Answer from the drawing. Dimensions are ordinates in mm from the lowest x, y and z of the part. Coordinates: 2 decimals unless noted, no trailing zeros. Write each loop counter-clockwise with the first axis right and the second up, starting at its lowest first coordinate (ties: lowest second). Pieces come first, ordered by that corner, then holes. Notation, with made-up numbers: (-38.75, 56) -> (-27.75, 56) arc R13 cw to (-27.75, 61) -> close; hole circle Ø6 at (-16, -10). An arc over 180 degrees is marked (long way). Return JSON: item names as keys, results as strings.
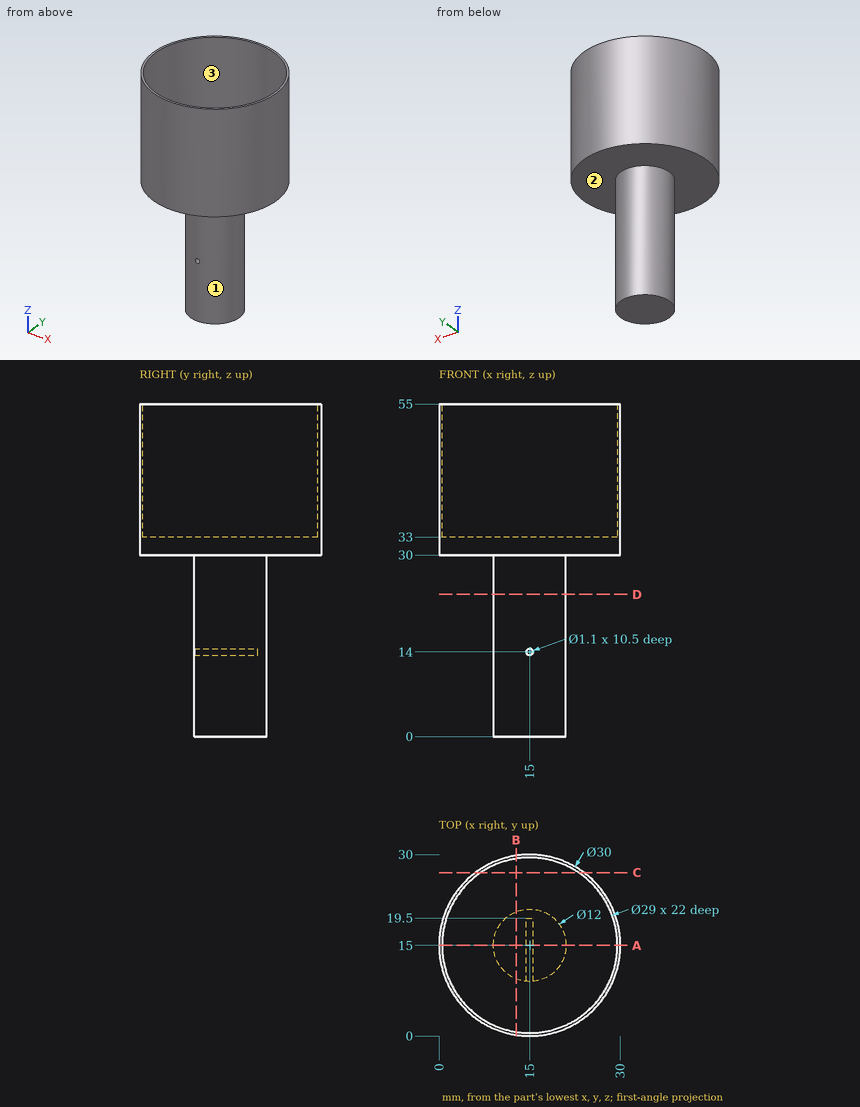
1. Consider L1, parallel to Y at x = 15, z = 37.5; L2, parallel to Z at x = 8.75, y = 4.5; L3, parallel to Z at x = 12.25, y = 18.75. Determine where each line is inside the solid, lowest interval first.
Taken from the geometry:
{"L1": "y = 0 to 0.5, 29.5 to 30", "L2": "z = 30 to 33", "L3": "z = 0 to 33"}
2. The part is cut by section B-B (x = 12.75). Determine the outline of the cut face in (y, z), then the cut area to 3 significant figures.
Taken from the geometry:
{"outline": "(0.17, 30) -> (9.44, 30) -> (9.44, 0) -> (20.56, 0) -> (20.56, 30) -> (29.83, 30) -> (29.83, 55) -> (29.32, 55) -> (29.32, 33) -> (0.68, 33) -> (0.68, 55) -> (0.17, 55) -> close", "area": "445 mm2"}
3. Flat-ended cylindrical pins translate along their axes: pin 1 Ø5 at (x, z) = (8.5, 47) entering from +Y; pin 2 Ø1 at (y, z) = (18.5, 14.5) entering from -X; pin 3 Ø3 at (x, y) = (8, 18.5) entering from +Z. Find the tip coordinate at first contact, or state that the pin passes through.
Taken from the geometry:
{"pin 1": "stops at y = 29.46", "pin 2": "stops at x = 9.8", "pin 3": "stops at z = 33"}
4. For a pull along X with two mould halves and no side action, classify the marked faces 1, 2 and 3 as +X half, -X half, draft (parallel to the pull), parting line (faces both ways), or undercut.
Taken from the geometry:
{"face 1": "parting line", "face 2": "draft", "face 3": "undercut"}
5. The part is cut by section A-A (y = 15). Determine the outline of the cut face in (x, z).
Taken from the geometry:
{"outline": "(0, 30) -> (9, 30) -> (9, 0) -> (21, 0) -> (21, 30) -> (30, 30) -> (30, 55) -> (29.5, 55) -> (29.5, 33) -> (0.5, 33) -> (0.5, 55) -> (0, 55) -> close; hole circle Ø1.1 at (15, 14)"}
6. The part is cut by section C-C (y = 27). Determine the outline of the cut face in (x, z).
Taken from the geometry:
{"outline": "(6, 30) -> (24, 30) -> (24, 55) -> (23.14, 55) -> (23.14, 33) -> (6.86, 33) -> (6.86, 55) -> (6, 55) -> close"}
7. The part is cut by section D-D (z = 23.5). Determine the outline of the cut face in (x, y).
Taken from the geometry:
{"outline": "circle Ø12 at (15, 15)"}
